Answer from the drawing. Dimensions are ordinates in mm from the lowest x, y and z of the part. Give positions to 0.01 mm unless a question says otherwise; leave off trailing zeros. Order: outer loops, then holes, each group sorted by start corner. A loop starts at its lowest first (then second) coordinate and runs counter-clockwise, first axis right, second up.
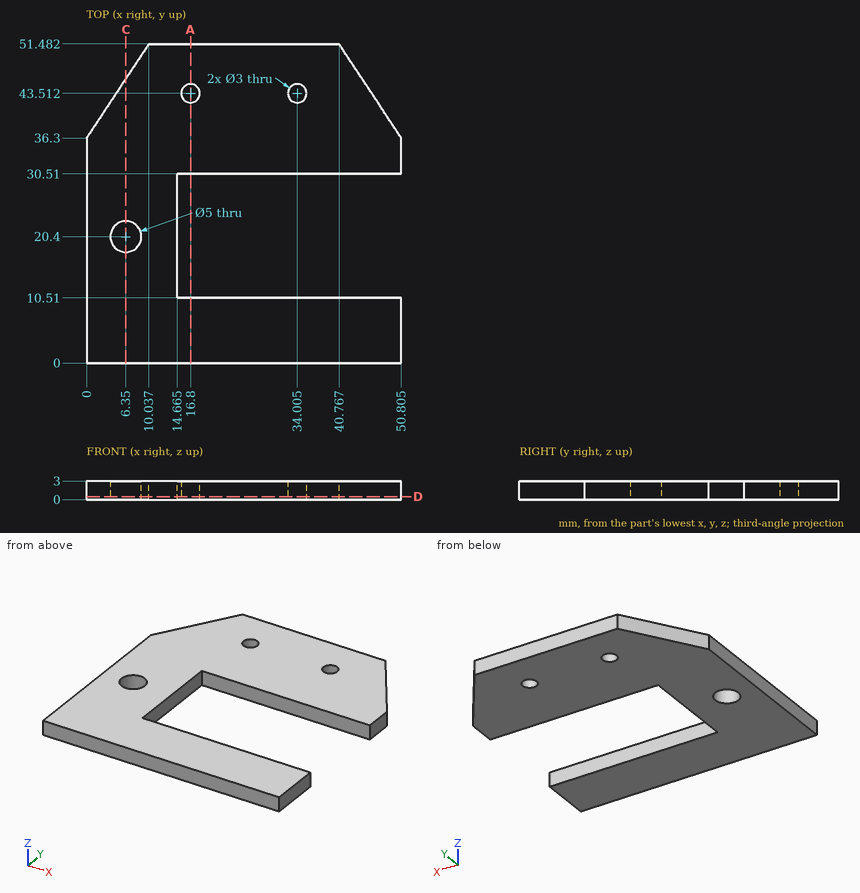
1) Consider L1, parallel to Y at x = 16.8, z = 1.65; L2, parallel to Y at x = 25, z = 0.3; L3, parallel to Y at x = 6.35, z = 1.3 (1 decimal). Determine where each line is inside the solid, lowest interval first.
Final values:
L1: y = 0 to 10.51, 30.51 to 42.01, 45.01 to 51.48
L2: y = 0 to 10.51, 30.51 to 51.48
L3: y = 0 to 17.9, 22.9 to 45.9
2) The part is cut by section C-C on x = 6.35. Determine the outline of the cut face in (y, z) (1 decimal), and give its area (3 significant figures).
Final values:
outline: (0, 0) - (17.9, 0) - (17.9, 3) - (0, 3) - close; (22.9, 0) - (45.9, 0) - (45.9, 3) - (22.9, 3) - close
area: 123 mm2
3) The part is cut by section A-A on x = 16.8. Determine the outline of the cut face in (y, z).
Final values:
outline: (0, 0) - (10.51, 0) - (10.51, 3) - (0, 3) - close; (30.51, 0) - (42.01, 0) - (42.01, 3) - (30.51, 3) - close; (45.01, 0) - (51.48, 0) - (51.48, 3) - (45.01, 3) - close
4) The part is cut by section D-D on z = 0.5. Count the separate pieces of the cut face and the enclosed holes in it, and give its area (3 significant figures).
Final values:
separate pieces: 1
enclosed holes: 3
area: 1,710 mm2
5) Given pin 1 (1.5 mm diameter, centred on y = 19.5, z = 1.5, fed in from +X) (1 decimal), flat-ended and moving along its own axis, determine where the tip first touches the part or whether it passes through.
Final values:
pin 1: stops at x = 14.7
